from build123d import *

# Parameters (mm, degrees)
F0_R           = 31.75
F1_DEPTH       = 9.525
F2_R           = 19.05
F3_DEPTH       = 25.4
F3_TAPER       = -30
F5_D           = 3.7973
F5_CSINK_D     = 7.7978
F5_CSINK_ANGLE = 82


with BuildPart() as f1:
    # F0 (on Top) → F1 (new body)
    with BuildSketch(Plane.XY):
        Circle(F0_R)
    extrude(amount=F1_DEPTH)

    # F2 (on face) → F3 (cut)
    with BuildSketch(Plane.XY.offset(9.525)):
        Circle(F2_R)
    extrude(amount=-F3_DEPTH, taper=F3_TAPER, mode=Mode.SUBTRACT)

    # F5 (through all)
    with Locations(Plane.XY.offset(9.525)):
        with Locations((-23.3718605846, 13.49375), (23.3718605846, 13.49375), (0, -26.9875)):
            CounterSinkHole(F5_D / 2, F5_CSINK_D / 2, counter_sink_angle=F5_CSINK_ANGLE)


solid = f1.part
Geometry check sheet. Reference: the model listing, model coordinates, mm. Round coordinates to 2 decimals unless told otherwise and drop trailing zeros. Order: outer loops, then holes, each group sorted by start corner. A loop starts at its lowest first (then second) coordinate and runs counter-clockwise, first axis right, second up. Notation, with made-up numbers: M -0.5,-6 L 12.5,-6 A18 ccw 12.5,21 Z; hole C 19.25,60 d1. An arc over 180 degrees is marked long. Answer in a Markdown table with one row per item.
(1) Scan lines: probe 1 along Y at (x, z) = (-6.5, 2.5); probe 2 along Y at (x, z) = (-4, 3.25); probe 3 along X at (y, z) = (-0.5, 7.75). Record each from-to range of solid material in increasing order. Write a range as from..to.
Responses:
| item | result |
|---|---|
| probe 1 | y = -31.08..-22.17, 22.17..31.08 |
| probe 2 | y = -31.5..-22.32, 22.32..31.5 |
| probe 3 | x = -31.75..-20.07, 20.07..31.75 |
(2) Go/stop test with flat-tipped pins: P1, Ø1.5, axis at y = 16, z = 2, coming from the -X side; P2, Ø2, axis at y = -4, z = 4.5, coming from the +X side; P3, Ø2, axis at y = 8, z = 7.5, coming from the +X side; P4, Ø2.5, axis at x = -23.37, y = 13.49, coming from the -Z side. Record where each tip stops, or that it passes through.
Responses:
| item | result |
|---|---|
| P1 | stops at x = -27.85 |
| P2 | stops at x = 31.61 |
| P3 | stops at x = 30.97 |
| P4 | passes through |
(3) Draft check along Y on faces 1 (the face through (-6.883, -30.995, 4.696)), 2 (the face through (19, 17, 0)), 3 (the face through (24.96, 12.28, 7.34)). Enter one of: released by +Y, released by -Y, zero draft, split by the parting line, or undercut.
Responses:
| item | result |
|---|---|
| face 1 | split by the parting line |
| face 2 | zero draft |
| face 3 | undercut |
(4) Sectioned sample at A-A, the plane x = 0. Record the cut outline in (y, z) (3 decimals).
Responses:
| item | result |
|---|---|
| outline | M -31.75,0 L -28.886,0 L -28.886,7.224 L -30.886,9.525 L -31.75,9.525 Z; M -25.089,0 L -24.549,0 L -19.05,9.525 L -23.089,9.525 L -25.089,7.224 Z; M 19.05,9.525 L 24.549,0 L 31.75,0 L 31.75,9.525 Z |
(5) Sectioned sample at B-B, the plane z = 5.75. Record the cut outline in (x, y), and give its area (3 significant figures).
Responses:
| item | result |
|---|---|
| outline | C 0,0 d63.5; hole C -23.37,13.49 d3.8; hole C 0,0 d42.46; hole C 0,-26.99 d3.8; hole C 23.37,13.49 d3.8 |
| area | 1,720 mm² |
